The model under review builds one solid part; all positions refer to its coordinate system, in mm. Round coordinates to 2 decimals unless told otherwise and drop trailing zeros. Write each loop counter-clockwise with the first axis right and the second up, starting at its lowest first coordinate (ties: lowest second). Pieces come first, ordered by that corner, then holes.
Item 1: Add section C-C (z = -0.05). Give the boundary of the cut face in (x, y) (3 decimals), plus the area to 3 significant figures.
Item 2: Add section D-D (y = -1.25). Give the boundary of the cut face in (x, z), plus the area to 3 significant figures.
Item 3: To check wall thickness, follow L1, parallel to Z at x = -0.25, y = 4; L2, parallel to Y at x = -0.3, z = 0.4. State the ranges of each line that lie inside material, in increasing order.
Item 4: Add section B-B (x = 0). Give the boundary of the cut face in (y, z) (3 decimals), plus the area to 3 significant figures.
Item 5: Add section A-A (y = 4). Give the boundary of the cut face in (x, z).
Item 6: Clearance check with a flat-ended pin moving along its axis: pin 1 Ø0.5 at (x, z) = (0, 0) entering from +Y. State where the tip first meets the part, or that it passes through.
Autodesk Inventor part; units mm, degrees
ref_plane "YZ Plane" through (0, 0, 0) normal (1, 0, 0) x (0, 1, 0)
ref_plane "XZ Plane" through (0, 0, 0) normal (0, 1, 0) x (-1, 0, 0)
ref_plane "XY Plane" through (0, 0, 0) normal (0, 0, 1) x (1, 0, 0)
sketch "Sketch1" plane through (0, 0, 0) normal (0, 1, 0) x (-1, 0, 0)
  line L0 (-0.5, 0.5) -> (0.5, 0.5)
  line L1 (0.5, 0.5) -> (0.5, -0.5)
  line L2 (0.5, -0.5) -> (-0.5, -0.5)
  line L3 (-0.5, -0.5) -> (-0.5, 0.5)
  line L4 (-0.5, 0.5) -> (0.5, -0.5) construction
  line L5 (0.5, 0.5) -> (-0.5, -0.5) construction
  point P0 (0, 0)
  dimension "d0" = 1
  dimension "d1" = 1
extrude "Extrusion1" add sketch "Sketch1" along normal blind 6.23
sketch "Sketch2" plane through (0, 0, 0) normal (0, -1, 0) x (1, 0, 0)
  line L0 (-0.32, 0.32) -> (0.32, 0.32)
  line L1 (0.32, 0.32) -> (0.32, -0.32)
  line L2 (0.32, -0.32) -> (-0.32, -0.32)
  line L3 (-0.32, -0.32) -> (-0.32, 0.32)
  line L4 (-0.32, 0.32) -> (0.32, -0.32) construction
  line L5 (0.32, 0.32) -> (-0.32, -0.32) construction
  point P0 (0, 0)
  dimension "d4" = 0.64
  dimension "d5" = 0.64
extrude "Extrusion2" add sketch "Sketch2" along normal blind 3.2
chamfer "Chamfer1" distance 0.155 angle 45 4 edges at (0, -3.2, 0.32) (0.32, -3.2, 0) (0, -3.2, -0.32) (-0.32, -3.2, 0)
sketch "Sketch3" plane through (0, 6.23, 0) normal (0, 1, 0) x (1, 0, 0)
  line L0 (0.32, 0.32) -> (-0.32, 0.32)
  line L1 (-0.32, 0.32) -> (-0.32, -0.32)
  line L2 (-0.32, -0.32) -> (0.32, -0.32)
  line L3 (0.32, -0.32) -> (0.32, 0.32)
  line L4 (0.32, 0.32) -> (-0.32, -0.32) construction
  line L5 (-0.32, 0.32) -> (0.32, -0.32) construction
  point P0 (0, 0)
  dimension "d11" = 0.64
  dimension "d12" = 0.64
extrude "Extrusion3" cut sketch "Sketch3" against normal blind 6
properties part number "pin" material "Gold"
Numbers:
1. outline: (-0.5, 0) - (-0.32, 0) - (-0.32, -3.045) - (-0.165, -3.2) - (0.165, -3.2) - (0.32, -3.045) - (0.32, 0) - (0.5, 0) - (0.5, 6.23) - (0.32, 6.23) - (0.32, 0.23) - (-0.32, 0.23) - (-0.32, 6.23) - (-0.5, 6.23) - close
1. area: 4.41 mm2
2. outline: (-0.32, -0.32) - (0.32, -0.32) - (0.32, 0.32) - (-0.32, 0.32) - close
2. area: 0.410 mm2
3. L1: z = -0.5 to -0.32, 0.32 to 0.5
3. L2: y = 0 to 6.23
4. outline: (-3.2, -0.165) - (-3.045, -0.32) - (0, -0.32) - (0, -0.5) - (6.23, -0.5) - (6.23, -0.32) - (0.23, -0.32) - (0.23, 0.32) - (6.23, 0.32) - (6.23, 0.5) - (0, 0.5) - (0, 0.32) - (-3.045, 0.32) - (-3.2, 0.165) - close
4. area: 4.41 mm2
5. outline: (-0.5, -0.5) - (0.5, -0.5) - (0.5, 0.5) - (-0.5, 0.5) - close; hole (-0.32, -0.32) - (0.32, -0.32) - (0.32, 0.32) - (-0.32, 0.32) - close
6. pin 1: stops at y = 0.23
